Can you work these out from the model? Positions are in its coordinate system, mm. Face numbers are marked on the shaded views. A direction names the side the tool comes from. Round coordinates to 2 decimals unless told otherwise and drop trailing zeros. Loops run counter-clockwise (first coordinate to the right, second up) from the corner with the lowest first, then second, coordinate; pieces in that order, holes last. Notation, with made-up numbers: (-9, 76.5) -> (18, 76.5) arc R26 ccw to (18, 91.5) -> close; hole circle Ø4 at (4.25, 13). An arc over 180 degrees is marked (long way). Use a Markdown table: item, result.
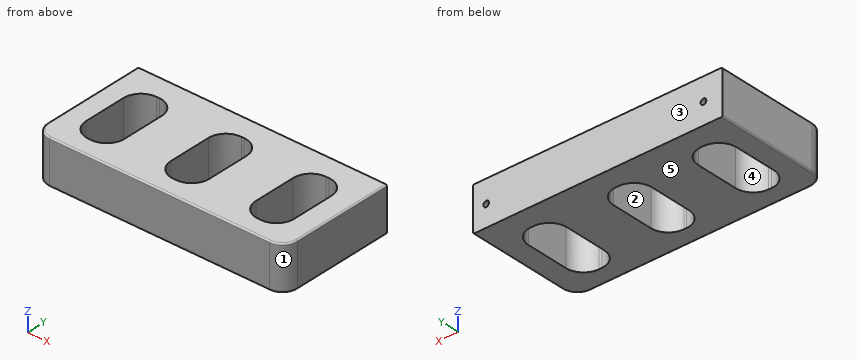
from build123d import *

# Parameters (mm, degrees)
F0_W     = 170
F0_H     = 80
F0_W_2   = 26
F0_H_2   = 53
F1_DEPTH = 30
F2_R     = 10.0472084404
F3_R     = 12
F4_R     = 1
F5_R     = 1.95
F6_DEPTH = 20


with BuildPart() as f1:
    # F0 (on Top) → F1 (new body)
    with BuildSketch(Plane.XY):
        with Locations((-5.2488362789, -6.2499986589)):
            Rectangle(F0_W, F0_H)
        with Locations((-63.4411496222, -7.5576923192)):
            Rectangle(F0_W_2, F0_H_2, mode=Mode.SUBTRACT)
        with Locations((-5.6146496222, -7.5576923192)):
            Rectangle(F0_W_2, F0_H_2, mode=Mode.SUBTRACT)
        with Locations((52.2118503778, -7.5576923192)):
            Rectangle(F0_W_2, F0_H_2, mode=Mode.SUBTRACT)
    extrude(amount=F1_DEPTH)

    # F2
    f2_edges = [f1.edges().sort_by_distance(p)[0] for p in [
        (-90.248836, -46.249999, 15),
        (79.751164, -46.249999, 15),
    ]]
    fillet(f2_edges, radius=F2_R)

    # F3
    f3_edges = [f1.edges().sort_by_distance(p)[0] for p in [
        (-50.44115, 18.942308, 15),
        (7.38535, 18.942308, 15),
        (65.21185, 18.942308, 15),
        (-76.44115, 18.942308, 15),
        (-18.61465, 18.942308, 15),
        (39.21185, 18.942308, 15),
        (39.21185, -34.057692, 15),
        (-18.61465, -34.057692, 15),
        (-76.44115, -34.057692, 15),
        (-50.44115, -34.057692, 15),
        (7.38535, -34.057692, 15),
        (65.21185, -34.057692, 15),
    ]]
    fillet(f3_edges, radius=F3_R)

    # F4
    f4_edges = [f1.edges().sort_by_distance(p)[0] for p in [
        (-90.248836, -1.226394, 30),
        (-87.306077, -43.307239, 30),
        (79.751164, -1.226394, 0),
    ]]
    fillet(f4_edges, radius=F4_R)

    # F5 (on face) → F6 (cut)
    with BuildSketch(Plane(origin=(0, 33.7500013411, 0), x_dir=(-1, 0, 0), z_dir=(0, 1, 0))):
        with Locations((-70.7511637211, 14.5192313939)):
            Circle(F5_R)
        with Locations((77.2488362789, 14.5192313939)):
            Circle(F5_R)
    extrude(amount=-F6_DEPTH, mode=Mode.SUBTRACT)


solid = f1.part
1. I need wall thicknesses on line 1 (X direction, y = -15, z = 5.25); line 2 (Y direction, x = 52.5, z = 28.25); line 3 (X direction, y = 10, z = 24.75). Which ranges of each line are inside material? Lowest first, please.
Answer sheet:
| item | result |
|---|---|
| line 1 | x = -90.25 to -76.44, -50.44 to -18.61, 7.39 to 39.21, 65.21 to 79.75 |
| line 2 | y = -46.25 to -34.06, 18.94 to 33.75 |
| line 3 | x = -90.25 to -76.05, -50.84 to -18.22, 6.99 to 39.61, 64.82 to 79.75 |
2. I want a section at A-A (z = 5). State how many separate pieces and enclosed holes the cut face has, plus the area to 3 significant figures.
Answer sheet:
| item | result |
|---|---|
| separate pieces | 1 |
| enclosed holes | 3 |
| area | 9,790 mm² |
3. Which directions (+Z, -Z, +X, -X, +Y, -Y) give clear straight access to the entire face, cutting with the end or side of a thin tool? Please do the marked faces 1 and 2.
Answer sheet:
| item | result |
|---|---|
| face 1 | +Z, -Z, +X, -Y |
| face 2 | +Z, -Z |
4. Will these pins go through, and if not, where does the flat tip stop? pin 1 Ø4 at (x, y) = (-37, 1.5) entering from -Z; pin 2 Ø1.2 at (x, z) = (-78, 15.5) entering from +Y.
Answer sheet:
| item | result |
|---|---|
| pin 1 | stops at z = 0 |
| pin 2 | stops at y = 13.75 |
5. I want a section at B-B (y = 3.5). Please give me the cut outline in (x, z).
Answer sheet:
| item | result |
|---|---|
| outline | (-90.25, 1) arc R1 ccw to (-89.25, 0) -> (-76.44, 0) -> (-76.44, 30) -> (-89.25, 30) arc R1 ccw to (-90.25, 29) -> close; (-50.44, 0) -> (-18.61, 0) -> (-18.61, 30) -> (-50.44, 30) -> close; (7.39, 0) -> (39.21, 0) -> (39.21, 30) -> (7.39, 30) -> close; (65.21, 0) -> (78.75, 0) arc R1 ccw to (79.75, 1) -> (79.75, 29) arc R1 ccw to (78.75, 30) -> (65.21, 30) -> close |
6. If we mould it in two halves opening along Y, with no side actions, what happens to the marked faces 3, 4 and 5? For each: +Y half, -Y half, draft (parallel to the pull), parting line (faces both ways), or undercut.
Answer sheet:
| item | result |
|---|---|
| face 3 | +Y half |
| face 4 | undercut |
| face 5 | draft |
7. I want a section at D-D (y = -32). Please give me the cut outline in (x, z), plus the area to 3 significant figures.
Answer sheet:
| item | result |
|---|---|
| outline | (-90.25, 1) arc R1 ccw to (-89.25, 0) -> (-71.16, 0) -> (-71.16, 30) -> (-89.25, 30) arc R1 ccw to (-90.25, 29) -> close; (-55.72, 0) -> (-13.33, 0) -> (-13.33, 30) -> (-55.72, 30) -> close; (2.1, 0) -> (44.49, 0) -> (44.49, 30) -> (2.1, 30) -> close; (59.93, 0) -> (78.75, 0) arc R1 ccw to (79.75, 1) -> (79.75, 29) arc R1 ccw to (78.75, 30) -> (59.93, 30) -> close |
| area | 3,710 mm² |
8. I want a section at C-C (x = 1.5). Please give me the cut outline in (y, z).
Answer sheet:
| item | result |
|---|---|
| outline | (-46.25, 1) arc R1 ccw to (-45.25, 0) -> (-32.38, 0) -> (-32.38, 30) -> (-45.25, 30) arc R1 ccw to (-46.25, 29) -> close; (17.27, 0) -> (33.75, 0) -> (33.75, 30) -> (17.27, 30) -> close |
